The model under review builds one solid part; all positions refer to its coordinate system, in mm. A direction names the side the tool comes from. Coordinates: 2 decimals unless noted, no trailing zeros. Order: outer loops, then holes, each group sorted by start corner. A loop starts at its lowest first (then second) coordinate and runs counter-clockwise, first axis right, second up. Notation, with made-up numbers: (-13.5, 74) -> (32.5, 74) arc R19 ccw to (32.5, 99) -> close; hole circle Ø7 at (86, 55.25). An arc over 180 degrees is marked (long way). Put each result on its own line as item: value.
from build123d import *

# Parameters (mm, degrees)
F0_W     = 101.6
F0_H     = 50.8
F1_DEPTH = 113.03
F0_W_2   = 72.39
F0_H_2   = 25.4
F2_DEPTH = 6.35
F3_W     = 44.45
F3_H     = 4.318
F4_DEPTH = 2.54
F5_W     = 11.43
F5_H     = 3.175
F6_DEPTH = 63.5
F7_W     = 2.286
F7_H     = 3.175
F8_DEPTH = 63.5


with BuildPart() as f1:
    # F0 (on Top) → F1 (new body)
    with BuildSketch(Plane.XY):
        with BuildLine():
            ThreePointArc((53.34, 25.4), (52.5960512242, 27.1960512242), (50.8, 27.94))
            Line((50.8, 27.94), (-50.8, 27.94))
            ThreePointArc((-50.8, 27.94), (-52.5960512242, 27.1960512242), (-53.34, 25.4))
            Line((-53.34, 25.4), (-53.34, -25.4))
            ThreePointArc((-53.34, -25.4), (-52.5960512242, -27.1960512242), (-50.8, -27.94))
            Line((-50.8, -27.94), (50.8, -27.94))
            ThreePointArc((50.8, -27.94), (52.5960512242, -27.1960512242), (53.34, -25.4))
            Line((53.34, -25.4), (53.34, 25.4))
        make_face()
        Rectangle(F0_W, F0_H, mode=Mode.SUBTRACT)
    extrude(amount=F1_DEPTH)

    # F0 (on Top) → F2 (join)
    with BuildSketch(Plane.XY):
        with BuildLine():
            ThreePointArc((53.34, 25.4), (52.5960512242, 27.1960512242), (50.8, 27.94))
            Line((50.8, 27.94), (-50.8, 27.94))
            ThreePointArc((-50.8, 27.94), (-52.5960512242, 27.1960512242), (-53.34, 25.4))
            Line((-53.34, 25.4), (-53.34, -25.4))
            ThreePointArc((-53.34, -25.4), (-52.5960512242, -27.1960512242), (-50.8, -27.94))
            Line((-50.8, -27.94), (50.8, -27.94))
            ThreePointArc((50.8, -27.94), (52.5960512242, -27.1960512242), (53.34, -25.4))
            Line((53.34, -25.4), (53.34, 25.4))
        make_face()
        Rectangle(F0_W, F0_H, mode=Mode.SUBTRACT)
        Rectangle(F0_W, F0_H)
        with Locations((6.985, -4.826)):
            Rectangle(F0_W_2, F0_H_2, mode=Mode.SUBTRACT)
    extrude(amount=F2_DEPTH)

    # F3 (on face) → F4 (cut)
    with BuildSketch(Plane.XY.offset(6.35)):
        with Locations((20.955, 10.033)):
            Rectangle(F3_W, F3_H)
    extrude(amount=-F4_DEPTH, mode=Mode.SUBTRACT)

    # F5 (on face) → F6 (join)
    with BuildSketch(Plane.XY.offset(6.35)):
        with Locations((-45.085, 5.3975)):
            Rectangle(F5_W, F5_H)
        with Locations((-45.085, 0.1905)):
            Rectangle(F5_W, F5_H)
    extrude(amount=F6_DEPTH)

    # F7 (on face) → F8 (join)
    with BuildSketch(Plane.XY.offset(6.35)):
        with Locations((49.657, 5.3975)):
            Rectangle(F7_W, F7_H)
        with Locations((49.657, 0.1905)):
            Rectangle(F7_W, F7_H)
    extrude(amount=F8_DEPTH)


solid = f1.part
Item 1: For pin 1 Ø5 at (x, y) = (41, 12.5) entering from +Z; pin 2 Ø15 at (x, y) = (23, -9) entering from +Z, all flat-tipped, find the tip position at first contact; note any pin that passes through.
Answers below:
pin 1: z = 6.35
pin 2: through
Item 2: Consider section A-A on z = 22. Write out the cut boundary in (x, y) (3 decimals).
Answers below:
outline: (-53.34, -25.4) arc R2.54 ccw to (-50.8, -27.94) -> (50.8, -27.94) arc R2.54 ccw to (53.34, -25.4) -> (53.34, 25.4) arc R2.54 ccw to (50.8, 27.94) -> (-50.8, 27.94) arc R2.54 ccw to (-53.34, 25.4) -> close; hole (-50.8, -25.4) -> (50.8, -25.4) -> (50.8, -1.397) -> (48.514, -1.397) -> (48.514, 1.778) -> (50.8, 1.778) -> (50.8, 3.81) -> (48.514, 3.81) -> (48.514, 6.985) -> (50.8, 6.985) -> (50.8, 25.4) -> (-50.8, 25.4) -> (-50.8, 6.985) -> (-39.37, 6.985) -> (-39.37, 3.81) -> (-50.8, 3.81) -> (-50.8, 1.778) -> (-39.37, 1.778) -> (-39.37, -1.397) -> (-50.8, -1.397) -> close
Item 3: Mouldability with a two-part tool opening along X and no side actions: class faces 4 (the flat face through (-1, 13, 0)), 5 (the flat face through (-39.37, 0, 38)), 6 (the cylindrical face through (-52.576, 27.216, 55.724)) as +X half, -X half, draft (parallel to the pull), parting line (faces both ways), or undercut.
Answers below:
face 4: draft
face 5: undercut
face 6: -X half
Item 4: Consider section B-B on x = 40. Write out the cut boundary in (y, z), and give its area (3 significant figures).
Answers below:
outline: (-27.94, 0) -> (-17.53, 0) -> (-17.53, 6.35) -> (-25.4, 6.35) -> (-25.4, 113.03) -> (-27.94, 113.03) -> close; (7.87, 0) -> (27.94, 0) -> (27.94, 113.03) -> (25.4, 113.03) -> (25.4, 6.35) -> (12.19, 6.35) -> (12.19, 3.81) -> (7.87, 3.81) -> close
area: 725 mm^2
Item 5: For faces 1 (the flat face through (-2, 7.874, 2)), 2 (the cylindrical face through (52.576, -27.216, 55.724)), 3 (the flat face through (48.514, 5, 38)), list the 3-axis set-ups (+Z, -Z, +X, -X, +Y, -Y) from which the entire face can be reached by the end or side of a thin tool; tool diameter is ignored.
Answers below:
face 1: +Z, -Z
face 2: +Z, -Z, +X, -Y
face 3: +Z
Item 6: For line 1 (Y direction, x = 11, z = 101); line 2 (X direction, y = 10, z = 98); line 3 (Z direction, x = -27, y = -25), list the stretches that pass through material, from the lowest coordinate up. Write a range as from..to.
Answers below:
line 1: -27.94..-25.4, 25.4..27.94
line 2: -53.34..-50.8, 50.8..53.34
line 3: 0..6.35
Item 7: Consider section D-D on x = -32.5. Write out the cut boundary in (y, z).
Answers below:
outline: (-27.94, 0) -> (27.94, 0) -> (27.94, 113.03) -> (25.4, 113.03) -> (25.4, 6.35) -> (-25.4, 6.35) -> (-25.4, 113.03) -> (-27.94, 113.03) -> close
Item 8: Consider section C-C on y = -5. Write out the cut boundary in (x, z), and give its area (3 significant figures).
Answers below:
outline: (-53.34, 0) -> (-29.21, 0) -> (-29.21, 6.35) -> (-50.8, 6.35) -> (-50.8, 113.03) -> (-53.34, 113.03) -> close; (43.18, 0) -> (53.34, 0) -> (53.34, 113.03) -> (50.8, 113.03) -> (50.8, 6.35) -> (43.18, 6.35) -> close
area: 760 mm^2
